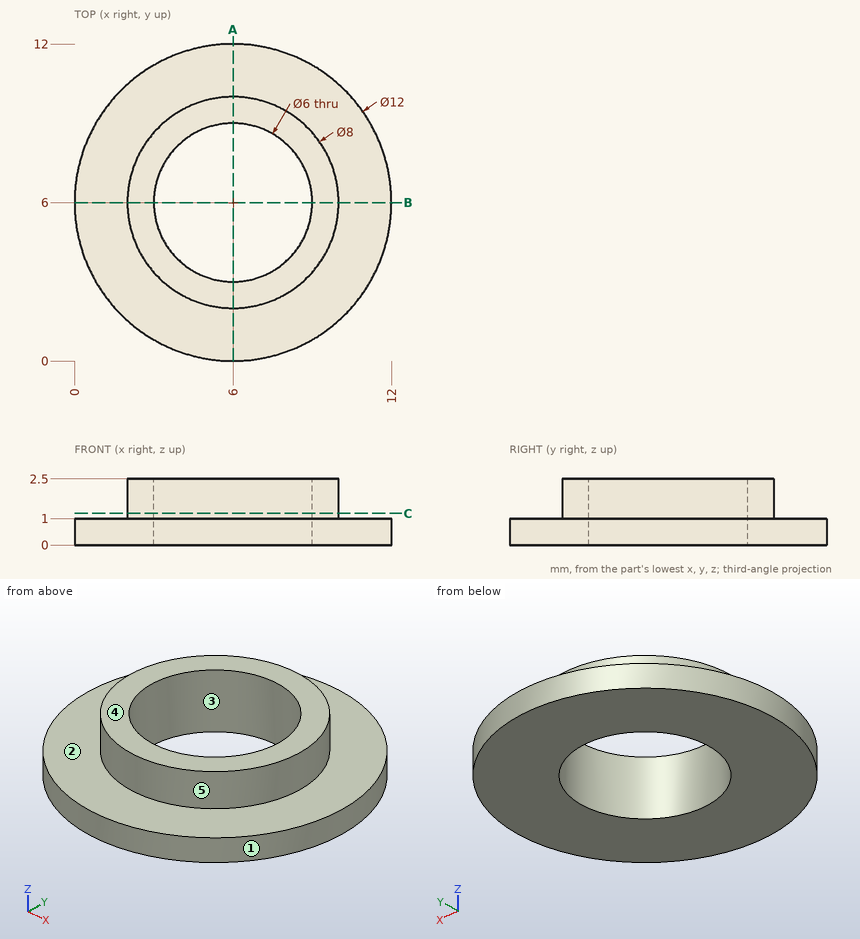
Can you work these out from the drawing? Everything is in mm from the part's minimum corner. A direction names the side the tool comes from. Round coordinates to 2 decimals unless told otherwise and drop trailing zeros. Loops run counter-clockwise (first coordinate to the right, second up) from the corner with the lowest first, then second, coordinate; pieces in that order, holes last. Notation, with made-up numbers: (54, 47) - (77, 47) arc R19 ccw to (77, 71) - close; hole circle Ø5 at (86.5, 10). An arc over 180 degrees is marked (long way). One line per question, with ' | ' between items. Start each with the question number.
Q1. For the marked faces 4 and 5, which set-ups out of +Z, -Z, +X, -X, +Y, -Y let a thin tool reach every point of the face, with its end or its side?
Q2. We'd pull the mould along X, two halves only. Please class the marked faces 1, 2 and 3: +X half, -X half, draft (parallel to the pull), parting line (faces both ways), or undercut.
Q3. I want a section at C-C (z = 1.2). Write out the boundary of the cut face in (x, y), then the cut area to 3 significant figures.
Q4. Will this pin go through, and if not, where does the flat tip stop? pin 1 (3.5 mm diameter, centred on x = 6, y = 6, fed in from +Z).
Q5. I want a section at A-A (x = 6). Write out the boundary of the cut face in (y, z).
Q6. Please list where these lines run through material, in increasing order: line 1 (Y direction, x = 6, z = 0.85); line 2 (Y direction, x = 6, z = 1.9); line 3 (Z direction, x = 1, y = 4.5). Write a range as [from, to].
Response values:
1) face 4: +Z, +X, -X, +Y, -Y | face 5: +Z
2) face 1: parting line | face 2: draft | face 3: undercut
3) outline: circle Ø8 at (6, 6); hole circle Ø6 at (6, 6) | area: 22.0 mm²
4) pin 1: passes through
5) outline: (0, 0) - (3, 0) - (3, 2.5) - (2, 2.5) - (2, 1) - (0, 1) - close; (9, 0) - (12, 0) - (12, 1) - (10, 1) - (10, 2.5) - (9, 2.5) - close
6) line 1: y = [0, 3], [9, 12] | line 2: y = [2, 3], [9, 10] | line 3: z = [0, 1]
